```python
from build123d import *

# Parameters (mm, degrees)
F0_R     = 3.175
F1_DEPTH = 3.048


with BuildPart() as f1:
    # F0 (on Front) → F1 (new body)
    with BuildSketch(Plane.XZ):
        with BuildLine():
            ThreePointArc((0, -7.9375), (5.6126600757, -5.6126600757), (7.9375, 0))
            ThreePointArc((7.9375, 0), (-0.4970693683, 7.9219207452), (-7.8752441368, -0.9921875))
            ThreePointArc((-7.8752441368, -0.9921875), (-5.2501627579, -5.953125), (0, -7.9375))
        make_face()
        Circle(F0_R, mode=Mode.SUBTRACT)
        with BuildLine():
            ThreePointArc((-7.8752441368, -0.9921875), (-0.4970693683, 7.9219207452), (7.9375, 0))
            Line((7.9375, 0), (36.5125, 0))
            ThreePointArc((36.5125, 0), (38.8373399243, 5.6126600757), (44.45, 7.9375))
            Line((44.45, 7.9375), (18.0149584735, 7.9375))
            ThreePointArc((18.0149584735, 7.9375), (12.0523084735, 10.6291369817), (10.127113946, 16.881475))
            Line((10.127113946, 16.881475), (15.7504882737, 61.515625))
            ThreePointArc((15.7504882737, 61.515625), (0, 47.625), (-15.7504882737, 61.515625))
            Line((-15.7504882737, 61.515625), (-7.8752441368, -0.9921875))
        make_face()
        with BuildLine():
            Line((36.5125, 0), (7.9375, 0))
            ThreePointArc((7.9375, 0), (5.6126600757, -5.6126600757), (0, -7.9375))
            Line((0, -7.9375), (44.45, -7.9375))
            ThreePointArc((44.45, -7.9375), (38.8373399243, -5.6126600757), (36.5125, 0))
        make_face()
        with BuildLine():
            ThreePointArc((44.45, 7.9375), (38.8373399243, 5.6126600757), (36.5125, 0))
            ThreePointArc((36.5125, 0), (38.8373399243, -5.6126600757), (44.45, -7.9375))
            ThreePointArc((44.45, -7.9375), (50.0626600757, -5.6126600757), (52.3875, 0))
            ThreePointArc((52.3875, 0), (50.0626600757, 5.6126600757), (44.45, 7.9375))
        make_face()
        with BuildLine():
            ThreePointArc((47.625, 0), (44.45, -3.175), (41.275, 0))
            ThreePointArc((41.275, 0), (44.45, 3.175), (47.625, 0))
        make_face(mode=Mode.SUBTRACT)
        with BuildLine():
            ThreePointArc((-15.7504882737, 65.484375), (-15.875, 63.5), (-15.7504882737, 61.515625))
            ThreePointArc((-15.7504882737, 61.515625), (0, 47.625), (15.7504882737, 61.515625))
            ThreePointArc((15.7504882737, 61.515625), (15.8438414904, 62.5058612634), (15.875, 63.5))
            ThreePointArc((15.875, 63.5), (15.8438414904, 64.4941387366), (15.7504882737, 65.484375))
            ThreePointArc((15.7504882737, 65.484375), (9.2504686451, 76.40133539), (-3.175, 79.0542598667))
            ThreePointArc((-3.175, 79.0542598667), (-11.6438383029, 74.2905817534), (-15.7504882737, 65.484375))
        make_face()
        with Locations((0, 63.5)):
            Circle(F0_R, mode=Mode.SUBTRACT)
        with BuildLine():
            Line((-9.4502929642, 115.490625), (-15.7504882737, 65.484375))
            ThreePointArc((-15.7504882737, 65.484375), (-11.6438383029, 74.2905817534), (-3.175, 79.0542598667))
            ThreePointArc((-3.175, 79.0542598667), (9.2504686451, 76.40133539), (15.7504882737, 65.484375))
            Line((15.7504882737, 65.484375), (9.4502929642, 115.490625))
            ThreePointArc((9.4502929642, 115.490625), (9.5063048942, 114.896483242), (9.525, 114.3))
            ThreePointArc((9.525, 114.3), (-0.596483242, 104.7936951058), (-9.4502929642, 115.490625))
        make_face()
        with BuildLine():
            ThreePointArc((0, 100.0252), (-0.9299359697, 97.7801359697), (-3.175, 96.8502))
            ThreePointArc((-3.175, 96.8502), (-5.4200640303, 102.2702640303), (0, 100.0252))
        make_face(mode=Mode.SUBTRACT)
        with BuildLine():
            ThreePointArc((9.4502929642, 115.490625), (0, 123.825), (-9.4502929642, 115.490625))
            ThreePointArc((-9.4502929642, 115.490625), (-0.596483242, 104.7936951058), (9.525, 114.3))
            ThreePointArc((9.525, 114.3), (9.5063048942, 114.896483242), (9.4502929642, 115.490625))
        make_face()
        with Locations((0, 114.3)):
            Circle(F0_R, mode=Mode.SUBTRACT)
    extrude(amount=F1_DEPTH)


solid = f1.part
```
Source: CAD feature listing. Evaluate the final solid. Frame: model axes, mm. A direction names the side the tool comes from. Coordinates: 2 decimals unless noted, no trailing zeros. Loops run counter-clockwise (first coordinate to the right, second up) from the corner with the lowest first, then second, coordinate; pieces in that order, holes last. Notation, with made-up numbers: (86.25, 76.5) -> (101.25, 76.5) arc R21 cw to (101.25, 92.5) -> close; hole circle Ø9 at (22, 42.5). An arc over 180 degrees is marked (long way). One line per item, written item: value. Start each with the question number.
Q1. Set-up query: faces 4 (the face through (3, -3.048, 59)), 5 (the face through (31, -2, 7.938)), 6 (the face through (12.9, -1.5, 38.9)). Return all of +Z, -Z, +X, -X, +Y, -Y with unobstructed straight access to the full face (end or side cutting, diameter ignored); none if empty.
Q2. Line query: line 1 along Z through (x, y) = (24.5, -0.25); line 2 along Z through (x, y) = (45.5, -0.95); line 3 along X through (y, z) = (-2.9, 116.5). Output: solid intervals per line, ascending.
Q3. Section query A-A, the plane y = -0.8. Give the number of separate pieces and of enclosed holes in the cut face, and give its area (3 significant figures).
Q4. Section query C-C, the plane x = 21. Return the cut outline in (y, z).
Q5. Section query B-B, the plane z = 114.3. Return the cut outline in (x, y) (3 decimals).
Q6. Mould query, pull axis X, two halves, no side actions, for faces 1 (the face through (-12.556, -1.503, 90.838)), 2 (the face through (1.707, -1.503, 66.177)), 3 (the face through (12.644, -1.503, 90.137)). Classes: pulls with the +X half, pulls with the -X half, needs draft (parallel to the pull), parting line crosses it, or undercut.
Q7. Contact query for flat-ended pins moving along their axis: P1, Ø5.5, axis at x = 0, z = 114.3, coming from the -Y side; P2, Ø1, axis at x = 26.5, y = -0.5, coming from the +Z side. Output: stop coordinate, or through.
Q8. Section query D-D, the plane z = 74.5. Return the cut outline in (x, y), and give its area (3 significant figures).
Results:
1. face 4: +Z, -Z, +X, -X, -Y
1. face 5: +Z, +X, +Y, -Y
1. face 6: +X, +Y, -Y
2. line 1: -7.94 to 7.94
2. line 2: -7.87 to -3, 3 to 7.87
2. line 3: -9.27 to -2.29, 2.29 to 9.27
3. separate pieces: 1
3. enclosed holes: 5
3. area: 3,610 mm^2
4. outline: (-3.05, -7.94) -> (0, -7.94) -> (0, 7.94) -> (-3.05, 7.94) -> close
5. outline: (-9.6, -3.048) -> (-3.175, -3.048) -> (-3.175, 0) -> (-9.6, 0) -> close; (3.175, -3.048) -> (9.6, -3.048) -> (9.6, 0) -> (3.175, 0) -> close
6. face 1: pulls with the -X half
6. face 2: undercut
6. face 3: pulls with the +X half
7. P1: through
7. P2: z = 7.94
8. outline: (-14.61, -3.05) -> (14.61, -3.05) -> (14.61, 0) -> (-14.61, 0) -> close
8. area: 89.1 mm^2
